```python
from build123d import *

# Parameters (mm, degrees)
SKETCH1_R               = 11
BOSS_EXTRUDE1_DEPTH     = 50
FILLET1_R               = 8
SKETCH2_R               = 11.5
SKETCH2_R_2             = 1.75
CUT_EXTRUDE1_DEPTH      = 10
SKETCH3_W               = 50
SKETCH3_H               = 5
BOSS_EXTRUDE2_DEPTH     = 50
SKETCH4_R               = 23.5
SKETCH4_R_2             = 2.25
CUT_EXTRUDE2_DEPTH      = 50
FILLET2_R               = 30
SKETCH6_R               = 2.25
CUT_EXTRUDE3_DEPTH      = 197
CUT_EXTRUDE3_DEPTH_BACK = 13
CUT_EXTRUDE4_DEPTH      = 3


with BuildPart() as part:
    # Sketch1 → Boss-Extrude1 (new body)
    with BuildSketch(Plane(origin=(0, 0, 0), x_dir=(1, 0, 0), z_dir=(0, 1, 0))):
        with BuildLine():
            Line((137.460581558, -14.5), (119.460581558, -14.5))
            Line((119.460581558, -14.5), (119.460581558, 10.5))
            Line((119.460581558, 10.5), (-24.539418442, 10.5))
            Line((-24.539418442, 10.5), (-24.539418442, -14.5))
            Line((-24.539418442, -14.5), (-42.539418442, -14.5))
            ThreePointArc((-42.539418442, -14.5), (-56.539418442, -0.5), (-42.539418442, 13.5))
            Line((-42.539418442, 13.5), (137.460581558, 13.5))
            ThreePointArc((137.460581558, 13.5), (151.460581558, -0.5), (137.460581558, -14.5))
        make_face()
        with Locations((-42.539418442, -0.5)):
            Circle(SKETCH1_R, mode=Mode.SUBTRACT)
        with Locations((137.460581558, -0.5)):
            Circle(SKETCH1_R, mode=Mode.SUBTRACT)
    extrude(amount=BOSS_EXTRUDE1_DEPTH)

    # Fillet1
    fillet1_edges = [part.edges().sort_by_distance(p)[0] for p in [
        (119.460581558, 25, 14.5),
        (-24.539418442, 25, 14.5),
    ]]
    fillet(fillet1_edges, radius=FILLET1_R)

    # Sketch2 → Cut-Extrude1 (cut)
    with BuildSketch(Plane.XY.offset(-10.5)):
        with Locations((0.460581558, 23)):
            Circle(SKETCH2_R)
        with Locations((15.960581558, 7.5)):
            Circle(SKETCH2_R_2)
        with Locations((-15.039418442, 7.5)):
            Circle(SKETCH2_R_2)
        with Locations((-15.039418442, 38.5)):
            Circle(SKETCH2_R_2)
        with Locations((15.960581558, 38.5)):
            Circle(SKETCH2_R_2)
        with Locations((78.960581558, 38.5)):
            Circle(SKETCH2_R_2)
        with Locations((109.960581558, 38.5)):
            Circle(SKETCH2_R_2)
        with Locations((109.960581558, 7.5)):
            Circle(SKETCH2_R_2)
        with Locations((94.460581558, 23)):
            Circle(SKETCH2_R)
        with Locations((78.960581558, 7.5)):
            Circle(SKETCH2_R_2)
    extrude(amount=-CUT_EXTRUDE1_DEPTH, mode=Mode.SUBTRACT)

    # Sketch3 → Boss-Extrude2 (add)
    with BuildSketch(Plane.XY.offset(-10.5)):
        with Locations((47.460581558, 47.5)):
            Rectangle(SKETCH3_W, SKETCH3_H)
    extrude(amount=BOSS_EXTRUDE2_DEPTH)

    # Sketch4 → Cut-Extrude2 (cut)
    with BuildSketch(Plane(origin=(0, 45, 0), x_dir=(-1, 0, 0), z_dir=(0, -1, 0))):
        with Locations((-47.460581558, -14.5)):
            Circle(SKETCH4_R)
        with Locations((-67.613124822, 5.652543264)):
            Circle(SKETCH4_R_2)
        with Locations((-27.308038294, 5.652543264)):
            Circle(SKETCH4_R_2)
        with Locations((-27.308038294, -34.652543264)):
            Circle(SKETCH4_R_2)
        with Locations((-67.613124822, -34.652543264)):
            Circle(SKETCH4_R_2)
    extrude(amount=-CUT_EXTRUDE2_DEPTH, mode=Mode.SUBTRACT)

    # Fillet2
    fillet2_edges = [part.edges().sort_by_distance(p)[0] for p in [
        (72.460581558, 47.5, -10.5),
        (22.460581558, 47.5, -10.5),
    ]]
    fillet(fillet2_edges, radius=FILLET2_R)

    # Sketch6 → Cut-Extrude3 (cut, two sides)
    with BuildSketch(Plane.ZY.offset(-139.460581558)) as cut_extrude3_sk:
        with Locations((0.5, 25)):
            Circle(SKETCH6_R)
    extrude(amount=CUT_EXTRUDE3_DEPTH, mode=Mode.SUBTRACT)
    extrude(cut_extrude3_sk.sketch, amount=-CUT_EXTRUDE3_DEPTH_BACK, mode=Mode.SUBTRACT)

    # Sketch7 → Cut-Extrude4 (cut)
    with BuildSketch(Plane(origin=(-24.539418442, 0, 0), x_dir=(0, 0, -1), z_dir=(1, 0, 0))):
        Polygon((-0.5, 20.843078062), (3.1, 22.921539031), (3.1, 27.078460969), (-0.5, 29.156921938), (-4.1, 27.078460969), (-4.1, 22.921539031), align=None)
    cut_extrude4 = extrude(amount=-CUT_EXTRUDE4_DEPTH, mode=Mode.SUBTRACT)

    # Mirror1: Cut-Extrude4 across plane
    add(cut_extrude4.mirror(Plane.ZY.offset(-47.460581558)), mode=Mode.SUBTRACT)


solid = part.part
```
Source: CAD feature listing. Evaluate the final solid. Frame: model axes, mm. A direction names the side the tool comes from. Give positions to 0.01 mm unless a question says otherwise; leave off trailing zeros. Write each loop counter-clockwise with the first axis right and the second up, starting at its lowest first coordinate (ties: lowest second). Pieces come first, ordered by that corner, then holes.
1. Access query for faces 1 (the face through (-14.23, 36.95, -11.98)), 2 (the face through (72.461, 47, 29)), 3 (the face through (121.87, 25.35, 12.22)). Directions: +Z, -Z, +X, -X, +Y, -Y. A direction counts if a zero-diameter tool reaches every point of the face in a straight line with its end or side. Return the directions, or none.
2. Material intervals for line 1 along Z through (x, y) = (100.5, 9.5); line 2 along X through (y, z) = (15, 12); line 3 along Z through (x, y) = (-28, 25), sorted ascending.
3. Pull-direction query (Y, two-part tool) for faces 4 (the face through (48, 0, -12)), 5 (the face through (17.577, 6.83, -11.979)), 6 (the face through (25.046, 47.465, 7.441)); classes: +Y half, -Y half, draft (parallel to the pull), parting line (faces both ways), or undercut.
4. First-contact query: pin 1 (1 mm diameter, centred on y = 35.5, z = -8, fed in from -X); pin 2 (4 mm diameter, centred on y = 46.5, z = 32, fed in from -X); pin 3 (3.5 mm diameter, centred on x = 120.5, y = 25, fed in from +Z); pin 4 (2.5 mm diameter, centred on y = 25, z = 0.5, fed in from +X). Flat tips, straight axial feed; report the tip coordinate or a pass-through.
5. Section query A-A (y = 17.5). Return the cut outline in (x, z), then the cut area to 3 significant figures.
Output values:
1. face 1: +Z, -Z
1. face 2: +Z, +X, +Y, -Y
1. face 3: +Z, +Y, -Y
2. line 1: z = -13.5 to -10.5
2. line 2: x = -50.52 to -26.73, 121.65 to 145.44
2. line 3: z = -13.5 to -1.75, 2.75 to 13.09
3. face 4: -Y half
3. face 5: undercut
3. face 6: draft
4. pin 1: stops at x = -54.03
4. pin 2: stops at x = 22.46
4. pin 3: stops at z = 12.57
4. pin 4: passes through
5. outline: (-42.54, -13.5) - (-9.64, -13.5) - (-9.64, -10.5) - (-24.54, -10.5) - (-24.54, 6.5) arc R8 ccw to (-32.54, 14.5) - (-42.54, 14.5) arc R14 ccw to start; (10.56, -13.5) - (84.36, -13.5) - (84.36, -10.5) - (10.56, -10.5) - close; (104.56, -13.5) - (137.46, -13.5) arc R14 ccw to (137.46, 14.5) - (127.46, 14.5) arc R8 ccw to (119.46, 6.5) - (119.46, -10.5) - (104.56, -10.5) - close; hole circle Ø22 at (-42.54, 0.5); hole circle Ø22 at (137.46, 0.5)
5. area: 1,150 mm2
